```python
from build123d import *

# Parameters (mm, degrees)
SKETCH1_R           = 13
SKETCH1_R_2         = 3.125
SKETCH1_R_3         = 5.5
SKETCH1_R_4         = 5.616805682
BOSS_EXTRUDE2_DEPTH = 13
SKETCH3_OUTSIDE_W   = 130.454
SKETCH3_OUTSIDE_H   = 128.254
CUT_EXTRUDE2_DEPTH  = 7
BOSS_EXTRUDE3_DEPTH = 3.5
BOSS_EXTRUDE4_DEPTH = 5
SKETCH6_R           = 4
BOSS_EXTRUDE5_DEPTH = 7


with BuildPart() as part:
    # Sketch1 → Boss-Extrude2 (new body, symmetric)
    with BuildSketch(Plane.XY):
        with BuildLine():
            ThreePointArc((45.332150622, 5.700536817), (48.696221254, 3.58439722), (49.999710802, -0.170057869))
            ThreePointArc((49.999710802, -0.170057869), (47.552825815, -15.450849719), (40.55057326, -29.251512923))
            ThreePointArc((40.55057326, -29.251512923), (37.289214732, -31.522758961), (33.323788774, -31.257400752))
            ThreePointArc((33.323788774, -31.257400752), (23.511410092, -32.360679775), (19.42993762, -41.351874493))
            ThreePointArc((19.42993762, -41.351874493), (18.456924262, -45.205218887), (15.289025708, -47.605101543))
            ThreePointArc((15.289025708, -47.605101543), (0, -50), (-15.289025708, -47.605101543))
            ThreePointArc((-15.289025708, -47.605101543), (-18.456924262, -45.205218887), (-19.42993762, -41.351874493))
            ThreePointArc((-19.42993762, -41.351874493), (-23.511410092, -32.360679775), (-33.323788774, -31.257400752))
            ThreePointArc((-33.323788774, -31.257400752), (-37.289214732, -31.522758961), (-40.55057326, -29.251512923))
            ThreePointArc((-40.55057326, -29.251512923), (-47.552825815, -15.450849719), (-49.999710802, -0.170057869))
            ThreePointArc((-49.999710802, -0.170057869), (-48.696221254, 3.58439722), (-45.332150622, 5.700536817))
            ThreePointArc((-45.332150622, 5.700536817), (-38.042260652, 12.360679775), (-40.025171716, 22.033738428))
            ThreePointArc((-40.025171716, 22.033738428), (-41.502926381, 25.72308243), (-40.350658246, 29.526672334))
            ThreePointArc((-40.350658246, 29.526672334), (-29.389262615, 40.450849719), (-15.612494996, 47.5))
            ThreePointArc((-15.612494996, 47.5), (-11.638995596, 47.420498199), (-8.586872248, 44.875))
            ThreePointArc((-8.586872248, 44.875), (0, 40), (8.586872248, 44.875))
            ThreePointArc((8.586872248, 44.875), (11.638995596, 47.420498199), (15.612494996, 47.5))
            ThreePointArc((15.612494996, 47.5), (29.389262615, 40.450849719), (40.350658246, 29.526672334))
            ThreePointArc((40.350658246, 29.526672334), (41.502926381, 25.72308243), (40.025171716, 22.033738428))
            ThreePointArc((40.025171716, 22.033738428), (38.042260652, 12.360679775), (45.332150622, 5.700536817))
        make_face()
        Circle(SKETCH1_R, mode=Mode.SUBTRACT)
        with Locations((0, -30)):
            Circle(SKETCH1_R_2, mode=Mode.SUBTRACT)
        with Locations((0, 30)):
            Circle(SKETCH1_R_2, mode=Mode.SUBTRACT)
        with Locations((22.335839587, 30.742645786)):
            Circle(SKETCH1_R_3, mode=Mode.SUBTRACT)
        with Locations((-22.335839587, 30.742645786)):
            Circle(SKETCH1_R_3, mode=Mode.SUBTRACT)
        with Locations((-36.140147619, -11.742645786)):
            Circle(SKETCH1_R_4, mode=Mode.SUBTRACT)
        with Locations((36.140147619, -11.742645786)):
            Circle(SKETCH1_R_4, mode=Mode.SUBTRACT)
    extrude(amount=BOSS_EXTRUDE2_DEPTH, both=True)

    # Sketch3 outside → Cut-Extrude2 (cut, symmetric)
    with BuildSketch(Plane.XY):
        with Locations((0, -1.1)):
            Rectangle(SKETCH3_OUTSIDE_W, SKETCH3_OUTSIDE_H)
        with BuildLine():
            Line((-12.93127555, -17.798373876), (-23.511410092, -32.360679775))
            ThreePointArc((-23.511410092, -32.360679775), (-20.283525766, -36.317381871), (-19.42993762, -41.351874493))
            ThreePointArc((-19.42993762, -41.351874493), (-18.456924262, -45.205218887), (-15.289025708, -47.605101543))
            ThreePointArc((-15.289025708, -47.605101543), (0, -50), (15.289025708, -47.605101543))
            ThreePointArc((15.289025708, -47.605101543), (18.456924262, -45.205218887), (19.42993762, -41.351874493))
            ThreePointArc((19.42993762, -41.351874493), (20.283525766, -36.317381871), (23.511410092, -32.360679775))
            Line((23.511410092, -32.360679775), (12.93127555, -17.798373876))
            ThreePointArc((12.93127555, -17.798373876), (0, 22), (-12.93127555, -17.798373876))
        make_face(mode=Mode.SUBTRACT)
    extrude(amount=CUT_EXTRUDE2_DEPTH, both=True, mode=Mode.SUBTRACT)



with BuildPart() as body_2:
    # Sketch4 → Boss-Extrude3 (new body, symmetric)
    with BuildSketch(Plane.XY):
        with BuildLine():
            Line((-5.187097318, -53.92545674), (-2.475294912, -105.639894327))
            ThreePointArc((-2.475294912, -105.639894327), (-2.120883278, -106.352371596), (-1.358533599, -106.580525999))
            ThreePointArc((-1.358533599, -106.580525999), (0, -106.5), (1.358533599, -106.580525999))
            ThreePointArc((1.358533599, -106.580525999), (2.120883278, -106.352371596), (2.475294912, -105.639894327))
            Line((2.475294912, -105.639894327), (5.187097318, -53.92545674))
            ThreePointArc((5.187097318, -53.92545674), (4.886610399, -53.157130414), (4.11095631, -52.876099336))
            ThreePointArc((4.11095631, -52.876099336), (0, -53.035665761), (-4.11095631, -52.876099336))
            ThreePointArc((-4.11095631, -52.876099336), (-4.886610399, -53.157130414), (-5.187097318, -53.92545674))
        make_face()
    extrude(amount=BOSS_EXTRUDE3_DEPTH, both=True)


with BuildPart() as part_1:
    add(part.part)

    add(body_2.part)  # Boss-Extrude4 merges body 2
    # Sketch5 → Boss-Extrude4 (add, symmetric)
    with BuildSketch(Plane.XY):
        with BuildLine():
            ThreePointArc((8.94, -49.194272024), (0, -50), (-8.94, -49.194272024))
            Line((-8.94, -49.194272024), (-5.63, -112.316418383))
            ThreePointArc((-5.63, -112.316418383), (0, -110), (5.63, -112.316418383))
            Line((5.63, -112.316418383), (8.94, -49.194272024))
        make_face()
        with BuildLine():
            Line((-2.475294912, -105.639894327), (-5.187097318, -53.92545674))
            ThreePointArc((-5.187097318, -53.92545674), (-4.886610399, -53.157130414), (-4.11095631, -52.876099336))
            ThreePointArc((-4.11095631, -52.876099336), (0, -53.035665761), (4.11095631, -52.876099336))
            ThreePointArc((4.11095631, -52.876099336), (4.886610399, -53.157130414), (5.187097318, -53.92545674))
            Line((5.187097318, -53.92545674), (2.475294912, -105.639894327))
            ThreePointArc((2.475294912, -105.639894327), (2.120883278, -106.352371596), (1.358533599, -106.580525999))
            ThreePointArc((1.358533599, -106.580525999), (0, -106.5), (-1.358533599, -106.580525999))
            ThreePointArc((-1.358533599, -106.580525999), (-2.120883278, -106.352371596), (-2.475294912, -105.639894327))
        make_face(mode=Mode.SUBTRACT)
    extrude(amount=BOSS_EXTRUDE4_DEPTH, both=True)

    # Sketch6 → Boss-Extrude5 (add, symmetric)
    with BuildSketch(Plane.XY):
        with BuildLine():
            ThreePointArc((5.63, -112.316418383), (0, -110), (-5.63, -112.316418383))
            ThreePointArc((-5.63, -112.316418383), (-3.078960864, -125.383765977), (8, -118))
            ThreePointArc((8, -118), (7.383765977, -114.921039136), (5.63, -112.316418383))
        make_face()
        with Locations((0, -118)):
            Circle(SKETCH6_R, mode=Mode.SUBTRACT)
    extrude(amount=BOSS_EXTRUDE5_DEPTH, both=True)


solid = part_1.part
```
Geometry check sheet. Reference: the model listing, model coordinates, mm. Give positions to 0.01 mm unless a question says otherwise; leave off trailing zeros. Order: outer loops, then holes, each group sorted by start corner. A loop starts at its lowest first (then second) coordinate and runs counter-clockwise, first axis right, second up.
1. Thickness scan on L1, parallel to Z at x = -1, y = 25.5; L2, parallel to Y at x = 0, z = 11.3 (3 decimals); L3, parallel to Z at x = 0, y = -110.5. Record the ranges inside material, lowest first.
2. Section check D-D, the plane y = -80. Enter the section's corners in (x, z), and give its area (3 significant figures).
3. Release check for a two-part mould opening along X. For faces 1 (the face through (25.29, 35.38, -10.04)), 2 (the face through (0.774, 21.986, 0.098)), 3 (the face through (-41.5, 25.7, 10)), 4 (the face through (-10, 10, 13)) record: pulls with the +X half, pulls with the -X half, needs draft (parallel to the pull), parting line crosses it, or undercut.
4. Section check C-C, the plane x = -35. Enter the section's corners in (y, z).
5. Section check A-A, the plane y = -8. Give the number of separate pieces and of enclosed holes in the cut face, and give its area (3 significant figures).
6. Gauge pin test, flat ends, axial feed: pin 1 Ø8 at (y, z) = (-95.5, -6) entering from +X; pin 2 Ø3 at (x, y) = (-1, -82) entering from -Z; pin 3 Ø9 at (x, y) = (0, -118) entering from -Z. Record the tip position at first contact, or that the pin passes through.
Values follow:
1. L1: z = -13 to -7, 7 to 13
1. L2: y = -50 to -33.125, -26.875 to -13, 13 to 26.875, 33.125 to 40
1. L3: z = -7 to 7
2. outline: (-7.32, -5) - (-3.82, -5) - (-3.82, -3.5) - (3.82, -3.5) - (3.82, -5) - (7.32, -5) - (7.32, 5) - (3.82, 5) - (3.82, 3.5) - (-3.82, 3.5) - (-3.82, 5) - (-7.32, 5) - close
2. area: 124 mm2
3. face 1: undercut
3. face 2: parting line crosses it
3. face 3: pulls with the -X half
3. face 4: needs draft
4. outline: (-31.7, -13) - (-17.24, -13) - (-17.24, -7) - (-31.7, -7) - close; (-31.7, 7) - (-17.24, 7) - (-17.24, 13) - (-31.7, 13) - close; (-6.24, -13) - (35.71, -13) - (35.71, -7) - (-6.24, -7) - close; (-6.24, 7) - (35.71, 7) - (35.71, 13) - (-6.24, 13) - close
5. separate pieces: 6
5. enclosed holes: 0
5. area: 1,020 mm2
6. pin 1: stops at x = 6.71
6. pin 2: stops at z = -3.5
6. pin 3: stops at z = -7
